```python
from build123d import *

# Parameters (mm, degrees)
SKETCH2_R          = 1.5
CUT_EXTRUDE1_DEPTH = 31


with BuildPart() as part:
    # Sketch1 → Revolve1 (revolve)
    with BuildSketch(Plane.XY, mode=Mode.PRIVATE) as revolve1_sk:
        Polygon((-1.5, -1.224136042), (-9.5, -1.224136042), (-9.5, 1.275863958), (-4, 1.275863958), (-4, 11.775863958), (-1.5, 11.775863958), align=None)
    revolve(revolve1_sk.sketch.rotate(Axis((0, -0.965665236, 0), (0, 1, 0)), 270), axis=Axis((0, -0.965665236, 0), (0, 1, 0)))

    # Sketch2 → Cut-Extrude1 (cut)
    with BuildSketch(Plane.XZ.offset(1.224136042)):
        with Locations(Location((-4.949747468, 4.949747468, 0), (0, 0, 270))):
            Circle(SKETCH2_R)
        with Locations(Location((4.949747468, 4.949747468, 0), (0, 0, 270))):
            Circle(SKETCH2_R)
        with Locations(Location((4.949747468, -4.949747468, 0), (0, 0, 270))):
            Circle(SKETCH2_R)
        with Locations(Location((-4.949747468, -4.949747468, 0), (0, 0, 270))):
            Circle(SKETCH2_R)
    extrude(amount=-CUT_EXTRUDE1_DEPTH, mode=Mode.SUBTRACT)


solid = part.part
```
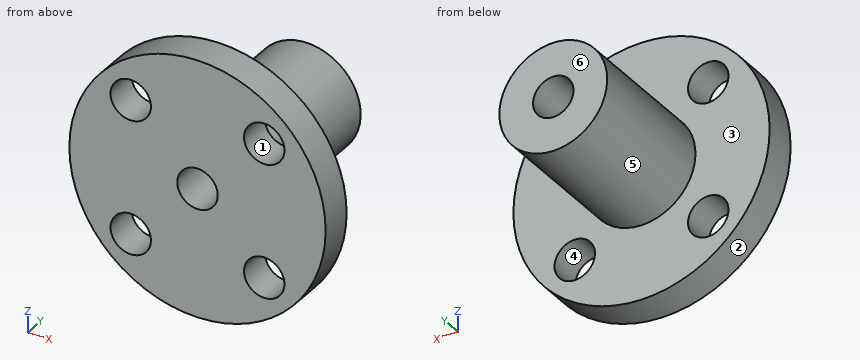
Check sheet for the modelled part. Datum: model origin and axes. Units: mm. Face numbers are marked on the shaded views. A direction names the side the tool comes from. Give positions to 0.01 mm unless a question says otherwise; leave off trailing zeros. Loops run counter-clockwise (first coordinate to the right, second up) from the corner with the lowest first, then second, coordinate; pieces in that order, holes last. Notation, with made-up numbers: M 75,38 L 91,38 A28 cw 91,72 Z; hole C 16,42 d3. An arc over 180 degrees is marked long. Answer as CSV lines item,"result".
Item 1: Sectioned sample at C-C, the plane x = 5.5. Enter the section's corners in (y, z).
Reply:
outline,"M -1.22,-7.75 L 1.28,-7.75 L 1.28,-6.35 L -1.22,-6.35 Z; M -1.22,-3.55 L 1.28,-3.55 L 1.28,3.55 L -1.22,3.55 Z; M -1.22,6.35 L 1.28,6.35 L 1.28,7.75 L -1.22,7.75 Z"
Item 2: Sectioned sample at D-D, the plane y = 0.25. Enter the section's corners in (x, z), then the cut area to 3 significant figures.
Reply:
outline,"C 0,0 d19; hole C -4.95,-4.95 d3; hole C -4.95,4.95 d3; hole C 0,0 d3; hole C 4.95,-4.95 d3; hole C 4.95,4.95 d3"
area,"248 mm^2"
Item 3: Scan lines: L1, parallel to X at y = 3.75, z = 0; L2, parallel to Z at x = 5.5, y = 1; L3, parallel to Y at x = -2.5, z = -4.5. Record each from-to range of solid material in increasing order.
Reply:
L1,"-4 to -1.5, 1.5 to 4"
L2,"-7.75 to -6.35, -3.55 to 3.55, 6.35 to 7.75"
L3,"-1.22 to 1.28"
Item 4: Sectioned sample at B-B, the plane x = 0. Enter the section's corners in (y, z), then the cut area to 3 significant figures.
Reply:
outline,"M -1.22,-9.5 L 1.28,-9.5 L 1.28,-4 L 11.78,-4 L 11.78,-1.5 L -1.22,-1.5 Z; M -1.22,1.5 L 11.78,1.5 L 11.78,4 L 1.28,4 L 1.28,9.5 L -1.22,9.5 Z"
area,"92.5 mm^2"
Item 5: Set-up check for the marked faces 5 and 6: record each of +Z, -Z, +X, -X, +Y, -Y from which the full face is reachable in a straight line by a thin tool's end or side.
Reply:
face 5,"+Y"
face 6,"+Z, -Z, +X, -X, +Y"
Item 6: Sectioned sample at A-A, the plane z = 0. Enter the section's corners in (x, y), then the cut area to 3 significant figures.
Reply:
outline,"M -9.5,-1.22 L -1.5,-1.22 L -1.5,11.78 L -4,11.78 L -4,1.28 L -9.5,1.28 Z; M 1.5,-1.22 L 9.5,-1.22 L 9.5,1.28 L 4,1.28 L 4,11.78 L 1.5,11.78 Z"
area,"92.5 mm^2"
Item 7: Depth check by flat-ended pin: pin 1 Ø1.8 at (x, z) = (0, 0) entering from -Y; pin 2 Ø6 at (x, z) = (6.5, -1.5) entering from +Y; pin 3 Ø5 at (x, y) = (-2.5, 7) entering from -Z; pin 4 Ø3.5 at (x, z) = (4.95, -4.95) entering from +Y. Enter the tip coordinate at first touch or a pass-through.
Reply:
pin 1,"through"
pin 2,"y = 11.78"
pin 3,"z = -4"
pin 4,"y = 1.28"
Item 8: Draft check along X on the marked faces 1, 2, 3 and 4. Enter one of: pulls with the +X half, pulls with the -X half, needs draft (parallel to the pull), parting line crosses it, or undercut.
Reply:
face 1,"undercut"
face 2,"parting line crosses it"
face 3,"needs draft"
face 4,"undercut"
